The drawing under review shows one solid part. Ordinate dimensions are in mm from its lowest x, y, z. Give positions to 0.01 mm unless a question says otherwise; leave off trailing zeros. Write each loop counter-clockwise with the first axis right and the second up, starting at its lowest first coordinate (ties: lowest second). Pieces come first, ordered by that corner, then holes. Notation, with made-up numbers: (-28, -7.75) -> (14, -7.75) arc R21 ccw to (14, -0.75) -> close; hole circle Ø5 at (75, 37.5). An arc over 180 degrees is marked (long way). Answer as a JSON object with one key per item and string values.
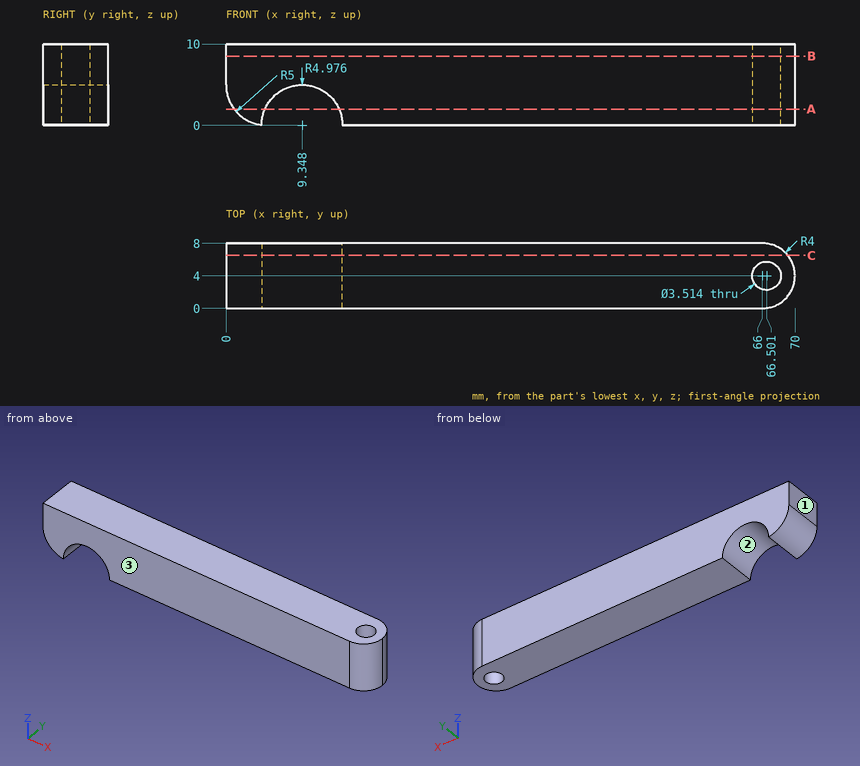
(1) We need section C-C, the plane y = 6.5. State the section outline as (x, z) points (1 decimal), then the cut area to 3 significant figures.
Here are the results:
{"outline": "(0, 5) arc R5 ccw to (4.4, 0) arc R5 cw to (14.3, 0) -> (69.1, 0) -> (69.1, 10) -> (0, 10) -> close", "area": "647 mm²"}
(2) The part is to be moulded in two halves that separate along X. For the marked faces 1, 2 and 3, say which applies: +X half, -X half, draft (parallel to the pull), parting line (faces both ways), or undercut.
Here are the results:
{"face 1": "-X half", "face 2": "undercut", "face 3": "draft"}
(3) We need section A-A, the plane z = 2. State the section outline as (x, y) points.
Here are the results:
{"outline": "(1, 0) -> (4.79, 0) -> (4.79, 8) -> (1, 8) -> close; (13.9, 0) -> (66, 0) arc R4 ccw to (66, 8) -> (13.9, 8) -> close; hole circle Ø3.51 at (66.5, 4)"}
(4) We need section B-B, the plane z = 8.5. State the section outline as (x, y) points.
Here are the results:
{"outline": "(0, 0) -> (66, 0) arc R4 ccw to (66, 8) -> (0, 8) -> close; hole circle Ø3.51 at (66.5, 4)"}
(5) Clearance check with flat-ended pins moving along their axes: pin 1 (3 mm diameter, centred on x = 66.5, y = 4, fed in from -Z); pin 2 (1 mm diameter, centred on y = 6.5, z = 1.5, fed in from -X). State where each tip first meets the part, or that it passes through.
Here are the results:
{"pin 1": "passes through", "pin 2": "stops at x = 1"}
(6) For line 1 along Y through (x, z) = (65.5, 8.5) (1 decimal); line 2 along Y through (x, z) = (66, 3.75) (1 decimal); line 3 along X through (y, z) = (3, 8.5) (1 decimal), list the stretches that pass through material, from the lowest coordinate up.
Here are the results:
{"line 1": "y = 0 to 2.6, 5.4 to 8", "line 2": "y = 0 to 2.3, 5.7 to 8", "line 3": "x = 0 to 65.1, 67.9 to 69.9"}
